Here's how the part is built. I have some questions about the finished solid (model axes, mm). A direction names the side the tool comes from. Coordinates: 2 decimals unless noted, no trailing zeros. Loops run counter-clockwise (first coordinate to the right, second up) from the corner with the lowest first, then second, coordinate; pieces in that order, holes last. Notation, with made-up numbers: (49.25, 59) -> (96.25, 59) arc R24 cw to (96.25, 73) -> close; hole circle Ø7 at (32, 78). An arc over 180 degrees is marked (long way). Answer as a JSON object with one key per item and string values. Group by question number.
Q1. I want a section at C-C on x = 64. Write out the boundary of the cut face in (y, z).
Q2. On a 3-axis mill with a long thin cutter (end or side, diameter ignored), from which of +Z, -Z, +X, -X, +Y, -Y can I reach the whole of each face in a straight line? I mean faces 1 (the flat face through (8, 0, 1)), 2 (the flat face through (52.1, -2, 1)), 3 (the flat face through (48, -8.1, 1)), 4 (the flat face through (75.9, -2, 1)), 5 (the flat face through (59.9, -10, 1)). Say none if no direction works.
Q3. I need wall thicknesses on line 1 (X direction, y = -2, z = 1.55); line 2 (X direction, y = -8.5, z = 0.7); line 3 (Y direction, x = 73.5, z = 2.5). Which ranges of each line are inside material? Lowest first, please.
Q4. I want a section at A-A on y = -2.25. Write out the boundary of the cut face in (x, z).
Q5. I'm going to push flat-ended pins straight in: pin 1 (1.5 mm diameter, centred on x = 2, z = 1.5, fed in from +Y); pin 2 (0.9 mm diameter, centred on y = -9.5, z = 1.5, fed in from -X); pin 3 (0.9 mm diameter, centred on y = -1, z = 1, fed in from +X). Where does each tip first touch, or does it pass through?
Q6. I want a section at B-B on y = -9.25. Write out the boundary of the cut face in (x, z), then the cut area to 3 significant figures.
```python
from build123d import *

# Parameters (mm, degrees)
SKETCH1_W           = 80
SKETCH1_H           = 11.2
BOSS_EXTRUDE1_DEPTH = 3
SKETCH3_W           = 20.2
SKETCH3_H           = 3.2
SKETCH3_W_2         = 4.2
SKETCH3_W_3         = 8.2
CUT_EXTRUDE1_DEPTH  = 4


with BuildPart() as part:
    # Sketch1 → Boss-Extrude1 (new body)
    with BuildSketch(Plane.XY):
        with Locations((40, -5.6)):
            Rectangle(SKETCH1_W, SKETCH1_H)
    extrude(amount=BOSS_EXTRUDE1_DEPTH)

    # Sketch3 → Cut-Extrude1 (cut, through all)
    with BuildSketch(Plane.XY):
        with Locations((10, -9.7)):
            Rectangle(SKETCH3_W, SKETCH3_H)
        with Locations((2, -1.5)):
            Rectangle(SKETCH3_W_2, SKETCH3_H)
        with Locations((32, -1.5)):
            Rectangle(SKETCH3_W_3, SKETCH3_H)
        with Locations((16, -1.5)):
            Rectangle(SKETCH3_W_3, SKETCH3_H)
        with Locations((48, -9.7)):
            Rectangle(SKETCH3_W_3, SKETCH3_H)
        with Locations((32, -9.7)):
            Rectangle(SKETCH3_W_3, SKETCH3_H)
        with Locations((70, -9.7)):
            Rectangle(SKETCH3_W, SKETCH3_H)
        with Locations((64, -1.5)):
            Rectangle(SKETCH3_W_3, SKETCH3_H)
        with Locations((48, -1.5)):
            Rectangle(SKETCH3_W_3, SKETCH3_H)
        with Locations((78, -1.5)):
            Rectangle(SKETCH3_W_2, SKETCH3_H)
    extrude(amount=CUT_EXTRUDE1_DEPTH, mode=Mode.SUBTRACT)


solid = part.part
```
Result set:
{
 "1": {"outline": "(-8.1, 0) -> (-3.1, 0) -> (-3.1, 3) -> (-8.1, 3) -> close"},
 "2": {"face 1": "+Z, -Z, +X, -X, +Y", "face 2": "+Z, -Z, +Y", "face 3": "+Z, -Z, -Y", "face 4": "+Z, -Z, +X, +Y", "face 5": "+Z, -Z, +X, -Y"},
 "3": {"line 1": "x = 4.1 to 11.9, 20.1 to 27.9, 36.1 to 43.9, 52.1 to 59.9, 68.1 to 75.9", "line 2": "x = 20.1 to 27.9, 36.1 to 43.9, 52.1 to 59.9", "line 3": "y = -8.1 to 0"},
 "4": {"outline": "(4.1, 0) -> (11.9, 0) -> (11.9, 3) -> (4.1, 3) -> close; (20.1, 0) -> (27.9, 0) -> (27.9, 3) -> (20.1, 3) -> close; (36.1, 0) -> (43.9, 0) -> (43.9, 3) -> (36.1, 3) -> close; (52.1, 0) -> (59.9, 0) -> (59.9, 3) -> (52.1, 3) -> close; (68.1, 0) -> (75.9, 0) -> (75.9, 3) -> (68.1, 3) -> close"},
 "5": {"pin 1": "stops at y = -3.1", "pin 2": "stops at x = 20.1", "pin 3": "stops at x = 75.9"},
 "6": {"outline": "(20.1, 0) -> (27.9, 0) -> (27.9, 3) -> (20.1, 3) -> close; (36.1, 0) -> (43.9, 0) -> (43.9, 3) -> (36.1, 3) -> close; (52.1, 0) -> (59.9, 0) -> (59.9, 3) -> (52.1, 3) -> close", "area": "70.2 mm²"}
}
